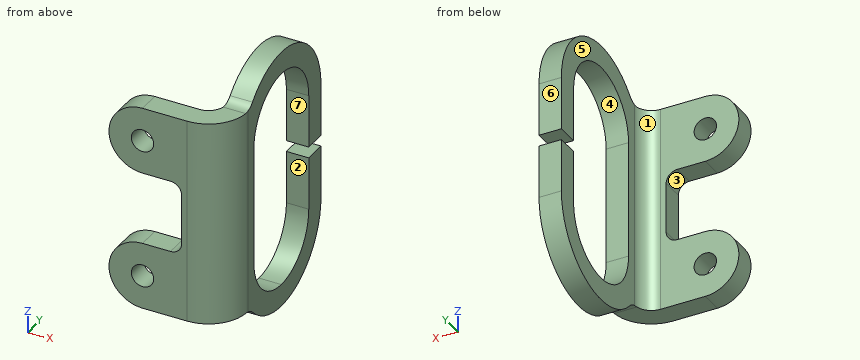
from build123d import *

# Parameters (mm, degrees)
SKETCH1_R           = 2
BOSS_EXTRUDE1_DEPTH = 4
SKETCH1_3_W         = 4
SKETCH1_3_H         = 18.5
SKETCH1_3_H_2       = 9.5
BOSS_EXTRUDE2_DEPTH = 35
FILLET3_R           = 2
CUT_EXTRUDE2_DEPTH  = 10
SKETCH4_W           = 2
SKETCH4_H           = 8.349248205
CUT_EXTRUDE3_DEPTH  = 10
FILLET4_R           = 3
FILLET6_R           = 3
FILLET5_R           = 7


with BuildPart() as part:
    # Sketch1 → Boss-Extrude1 (new body)
    with BuildSketch(Plane(origin=(0, 0, 0), x_dir=(1, 0, 0), z_dir=(0, 1, 0))):
        with BuildLine():
            Line((33.647984737, 18.5), (22.647984737, 18.5))
            ThreePointArc((22.647984737, 18.5), (16.647984737, 12.5), (22.647984737, 6.5))
            Line((22.647984737, 6.5), (29.647984737, 6.5))
            Line((29.647984737, 6.5), (29.647984737, -6.5))
            Line((29.647984737, -6.5), (22.647984737, -6.5))
            ThreePointArc((22.647984737, -6.5), (16.647984737, -12.5), (22.647984737, -18.5))
            Line((22.647984737, -18.5), (33.647984737, -18.5))
            Line((33.647984737, -18.5), (33.647984737, 18.5))
        make_face()
        with Locations((22.647984737, 12.5)):
            Circle(SKETCH1_R, mode=Mode.SUBTRACT)
        with Locations((22.647984737, -12.5)):
            Circle(SKETCH1_R, mode=Mode.SUBTRACT)
    extrude(amount=BOSS_EXTRUDE1_DEPTH)

    # Sketch1_3 → Boss-Extrude2 (add)
    with BuildSketch(Plane(origin=(0, 0, 0), x_dir=(1, 0, 0), z_dir=(0, 1, 0))):
        with Locations((35.647984737, 9.25)):
            Rectangle(SKETCH1_3_W, SKETCH1_3_H)
        with Locations((35.647984737, -9.25)):
            Rectangle(SKETCH1_3_W, SKETCH1_3_H)
        with Locations((35.647984737, 23.25)):
            Rectangle(SKETCH1_3_W, SKETCH1_3_H_2)
        with Locations((35.647984737, -23.25)):
            Rectangle(SKETCH1_3_W, SKETCH1_3_H_2)
    extrude(amount=BOSS_EXTRUDE2_DEPTH)

    # Fillet3
    fillet3_edges = [part.edges().sort_by_distance(p)[0] for p in [
        (29.647984737, 2, 6.5),
        (29.647984737, 2, -6.5),
    ]]
    fillet(fillet3_edges, radius=FILLET3_R)

    # Sketch3 → Cut-Extrude2 (cut)
    with BuildSketch(Plane(origin=(37.647984737, 0, 0), x_dir=(0, 0, -1), z_dir=(1, 0, 0))):
        with BuildLine():
            Line((-10.5, 9), (0, 9))
            Line((0, 9), (0, 18))
            Line((0, 18), (0, 27))
            Line((0, 27), (-10.5, 27))
            ThreePointArc((-10.5, 27), (-19.5, 18), (-10.5, 9))
        make_face()
        with BuildLine():
            Line((0, 18), (0, 9))
            Line((0, 9), (10.5, 9))
            ThreePointArc((10.5, 9), (16.863961031, 11.636038969), (19.5, 18))
            Line((19.5, 18), (0, 18))
        make_face()
        with BuildLine():
            Line((0, 27), (0, 18))
            Line((0, 18), (19.5, 18))
            ThreePointArc((19.5, 18), (16.863961031, 24.363961031), (10.5, 27))
            Line((10.5, 27), (0, 27))
        make_face()
        with BuildLine():
            Line((-28, 0), (-18.5, 0))
            Line((-18.5, 0), (-18.5, 7.753049234))
            ThreePointArc((-18.5, 7.753049234), (-22.792484695, 22.230226947), (-10.5, 31))
            Line((-10.5, 31), (0, 31))
            Line((0, 31), (0, 35))
            Line((0, 35), (-28, 35))
            Line((-28, 35), (-28, 0))
        make_face()
        with BuildLine():
            Line((18.5, 7.753049234), (18.5, 0))
            Line((18.5, 0), (28, 0))
            Line((28, 0), (28, 35))
            Line((28, 35), (0, 35))
            Line((0, 35), (0, 31))
            Line((0, 31), (10.5, 31))
            ThreePointArc((10.5, 31), (22.792484695, 22.230226947), (18.5, 7.753049234))
        make_face()
    extrude(amount=-CUT_EXTRUDE2_DEPTH, mode=Mode.SUBTRACT)

    # Sketch4 → Cut-Extrude3 (cut)
    with BuildSketch(Plane(origin=(37.647984737, 0, 0), x_dir=(0, 0, -1), z_dir=(1, 0, 0))):
        with Locations((0, 31.174624103)):
            Rectangle(SKETCH4_W, SKETCH4_H)
    extrude(amount=-CUT_EXTRUDE3_DEPTH, mode=Mode.SUBTRACT)

    # Fillet4
    fillet4_edges = [part.edges().sort_by_distance(p)[0] for p in [
        (35.647984737, 7.753049234, 18.5),
        (35.647984737, 7.753049234, -18.5),
    ]]
    fillet(fillet4_edges, radius=FILLET4_R)

    # Fillet6
    fillet6_edges = [part.edges().sort_by_distance(p)[0] for p in [
        (33.647984737, 4, 0),
    ]]
    fillet(fillet6_edges, radius=FILLET6_R)

    # Fillet5
    fillet5_edges = [part.edges().sort_by_distance(p)[0] for p in [
        (37.647984737, 0, 0),
    ]]
    fillet(fillet5_edges, radius=FILLET5_R)


solid = part.part
CAD build for the part. Positions are in the model's coordinates, mm. Face numbers are marked on the shaded views. A direction names the side the tool comes from. Coordinates: 2 decimals unless noted, no trailing zeros. Write each loop counter-clockwise with the first axis right and the second up, starting at its lowest first coordinate (ties: lowest second). Pieces come first, ordered by that corner, then holes. Notation, with made-up numbers: M 18,87.25 L 22,87.25 A22 cw 22,105.25 Z; hole C 60.5,-4.75 d8. An arc over 180 degrees is marked long. Return JSON: item names as keys, results as strings.
Item 1: Slice it at D-D, the plane x = 35.5. Write the cut outline in (y, z).
Findings below:
{"outline": "M 1.95,-18.5 L 6.38,-18.5 A3 cw 8.56,-19.44 A13 ccw 31,-10.5 L 31,-1 L 27,-1 L 27,-10.5 A9 cw 9,-10.5 L 9,10.5 A9 cw 27,10.5 L 27,1 L 31,1 L 31,10.5 A13 ccw 8.56,19.44 A3 cw 6.38,18.5 L 1.95,18.5 Z"}
Item 2: Slice it at A-A, the plane x = 25.5. Write the cut outline in (y, z).
Findings below:
{"outline": "M 0,-18.5 L 4,-18.5 L 4,-6.5 L 0,-6.5 Z; M 0,6.5 L 4,6.5 L 4,18.5 L 0,18.5 Z"}
Item 3: Which spindle directions (+Z, -Z, +X, -X, +Y, -Y) get a long thin tool onto all of the face, cutting with end or side? Do the marked faces 5, 6 and 7. Say none if no direction does.
Findings below:
{"face 5": "+Z, -Z, -X, +Y", "face 6": "+Z, -Z, +X, -X, +Y", "face 7": "+X, -X"}
Item 4: Probe line 1 (Y direction, x = 25.75, z = -7); line 2 (X direction, y = 8, z = -10); line 3 (Z direction, x = 35, y = 21). List the from-to ranges inside material, lowest first. Write a range as from..to.
Findings below:
{"line 1": "y = 0..4", "line 2": "x = 33.65..37.65", "line 3": "z = -23.15..-18.99, 18.99..23.15"}
Item 5: Slice it at C-C, the plane z = 10. Write the cut outline in (x, y).
Findings below:
{"outline": "M 17.19,0 L 30.65,0 A7 ccw 37.65,7 L 37.65,9 L 33.65,9 L 33.65,7 A3 cw 30.65,4 L 17.19,4 Z; M 33.65,27 L 37.65,27 L 37.65,31 L 33.65,31 Z"}
Item 6: Slice it at B-B, the plane y = 13. Write the cut outline in (x, z), and give its area (3 significant figures).
Findings below:
{"outline": "M 33.65,-22.5 L 37.65,-22.5 L 37.65,-17.98 L 33.65,-17.98 Z; M 33.65,17.98 L 37.65,17.98 L 37.65,22.5 L 33.65,22.5 Z", "area": "36.1 mm2"}
Item 7: Drop flat-ended pins along their axis: pin 1 Ø1.5 at (y, z) = (9.5, -18.5) entering from -X; pin 2 Ø4.5 at (x, y) = (35, 30) entering from +Z; pin 3 Ø3 at (y, z) = (3, 1.5) entering from -X. Give the stop position or say it passes through.
Findings below:
{"pin 1": "stops at x = 33.65", "pin 2": "stops at z = 19.1", "pin 3": "stops at x = 29.65"}
Item 8: Two-plate mould, pull along Y, no slides. Class the marked faces 1, 2, 3 and 4: +Y half, -Y half, draft (parallel to the pull), parting line (faces both ways), or undercut.
Findings below:
{"face 1": "+Y half", "face 2": "undercut", "face 3": "draft", "face 4": "undercut"}
